Design review of the part shown in the three views and the two pictorial views. Dimensions are in mm from the part's minimum x, y and z. A direction names the side the tool comes from. Round coordinates to 2 decimals unless told otherwise and drop trailing zeros. Loops run counter-clockwise (first coordinate to the right, second up) from the corner with the lowest first, then second, coordinate; pieces in that order, holes last. Notation, with made-up numbers: (47, 3) -> (101, 3) arc R23 cw to (101, 20) -> close; hole circle Ø11 at (13, 9.5). An arc over 180 degrees is marked (long way). Use a Markdown table: item, result. Add a question column.
1) Consider section B-B on x = 111.5. Give the boundary of the cut face in (y, z) (1 decimal), plus the area to 3 significant figures.
2) For the marked faces 1 and 2, list the 3-axis set-ups (+Z, -Z, +X, -X, +Y, -Y) from which the entire face can be reached by the end or side of a thin tool; tool diameter is ignored.
3) Consider section C-C on y = 20. Give the boundary of the cut face in (x, z) (3 decimals).
4) Consider section A-A on z = 102. Give the boundary of the cut face in (x, y) (3 decimals), plus the area to 3 significant figures.
5) Insertion check: pin 1 (1.5 mm diameter, centred on x = 82, z = 108, fed in from -Y); pin 2 (19 mm diameter, centred on x = 102.5, z = 100, fed in from +Y). Each pin has a flat end and moves straight along its axis. Give the tip position at first contact, or say it passes through.
6) Wall thickness on probe 1 along Z at (x, y) = (105, 21.75); probe 2 along Y at (x, z) = (108.5, 125.5) (3 decimals); probe 3 along Y at (x, z) = (96.5, 91.5): over which ranges is each line inside the solid? List them lowest first.
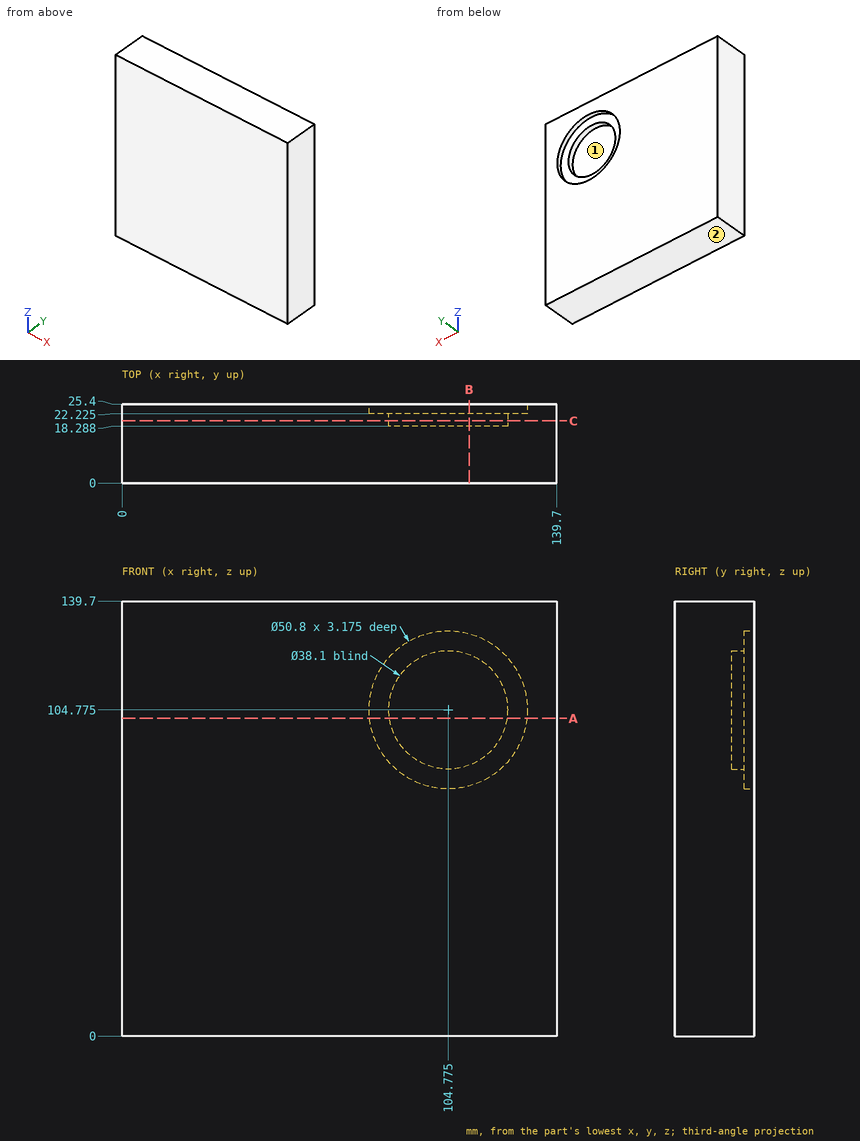
Result set:
| question | item | result |
|---|---|---|
| 1 | outline | (0, 0) -> (25.4, 0) -> (25.4, 80.3) -> (22.2, 80.3) -> (22.2, 87) -> (18.3, 87) -> (18.3, 122.6) -> (22.2, 122.6) -> (22.2, 129.3) -> (25.4, 129.3) -> (25.4, 139.7) -> (0, 139.7) -> close |
| 1 | area | 3,250 mm2 |
| 2 | face 1 | +Y |
| 2 | face 2 | -Z, +X, -X, +Y, -Y |
| 3 | outline | (0, 0) -> (139.7, 0) -> (139.7, 139.7) -> (0, 139.7) -> close; hole circle Ø38.1 at (104.775, 104.775) |
| 4 | outline | (0, 0) -> (139.7, 0) -> (139.7, 25.4) -> (130.023, 25.4) -> (130.023, 22.225) -> (123.622, 22.225) -> (123.622, 18.288) -> (85.928, 18.288) -> (85.928, 22.225) -> (79.527, 22.225) -> (79.527, 25.4) -> (0, 25.4) -> close |
| 4 | area | 3,240 mm2 |
| 5 | pin 1 | y = 0 |
| 5 | pin 2 | y = 18.29 |
| 6 | probe 1 | 0 to 85.73, 123.82 to 139.7 |
| 6 | probe 2 | 0 to 22.225 |
| 6 | probe 3 | 0 to 18.29 |
